from build123d import *

# Parameters (mm, degrees)
SKETCH1_W           = 135
SKETCH1_H           = 80
BOSS_EXTRUDE1_DEPTH = 40
SKETCH2_R           = 1.5
CUT_EXTRUDE1_DEPTH  = 10
SKETCH3_R           = 1.5
CUT_EXTRUDE2_DEPTH  = 10
CAVITY1_START       = 5.91875
CAVITY1_DEPTH       = 68.1625
CAVITY1_START_2     = 5
CAVITY1_2_DEPTH     = 125
SKETCH4_W           = 135
SKETCH4_H           = 25
CUT_EXTRUDE3_DEPTH  = 100


with BuildPart() as part:
    # Sketch1 → Boss-Extrude1 (new body)
    with BuildSketch(Plane.XY):
        with Locations((67.5, 40)):
            Rectangle(SKETCH1_W, SKETCH1_H)
    extrude(amount=-BOSS_EXTRUDE1_DEPTH)

    # Sketch2 → Cut-Extrude1 (cut)
    with BuildSketch(Plane(origin=(0, 0, -40), x_dir=(-1, 0, 0), z_dir=(0, 0, -1))):
        with Locations((-53.3, 40)):
            Circle(SKETCH2_R)
        with Locations((-53.3, 58.35)):
            Circle(SKETCH2_R)
        with Locations((-53.3, 21.65)):
            Circle(SKETCH2_R)
        with Locations((-23.3, 58.35)):
            Circle(SKETCH2_R)
        with Locations((-23.3, 40)):
            Circle(SKETCH2_R)
        with Locations((-23.3, 21.65)):
            Circle(SKETCH2_R)
        with Locations((-115.7, 40)):
            Circle(SKETCH2_R)
        with Locations((-115.7, 56)):
            Circle(SKETCH2_R)
        with Locations((-113.1, 61.75)):
            Circle(SKETCH2_R)
        with Locations((-113.1, 49.75)):
            Circle(SKETCH2_R)
        with Locations((-113.1, 18.25)):
            Circle(SKETCH2_R)
        with Locations((-113.1, 30.25)):
            Circle(SKETCH2_R)
    extrude(amount=-CUT_EXTRUDE1_DEPTH, mode=Mode.SUBTRACT)

    # Sketch3 → Cut-Extrude2 (cut)
    with BuildSketch(Plane.ZY):
        with Locations((-10, 54.05)):
            Circle(SKETCH3_R)
        with Locations((-10, 25.95)):
            Circle(SKETCH3_R)
        with Locations((-26, 40)):
            Circle(SKETCH3_R)
    extrude(amount=-CUT_EXTRUDE2_DEPTH, mode=Mode.SUBTRACT)

    # Cavity1: read off the stored shape, not the designer's step
    # Cavity1 outline → Cavity1 (cut)
    with BuildSketch(Plane(origin=(0, 0, 0), x_dir=(1, 0, 0), z_dir=(0, 1, 0)).offset(CAVITY1_START)):
        Polygon((128.3771626, 35.7), (6.6228374, 35.7), (5.688, 0), (129.312, 0), align=None)
    extrude(amount=CAVITY1_DEPTH, mode=Mode.SUBTRACT)

    # Cavity1 2 outline → Cavity1 2 (add)
    with BuildSketch(Plane.YZ.offset(CAVITY1_START_2)):
        Polygon((74.08125, 0), (73.141830064, -35.7), (74.08125, -35.7), align=None)
        Polygon((6.858169936, -35.7), (5.91875, 0), (5.91875, -35.7), align=None)
    extrude(amount=CAVITY1_2_DEPTH)

    # Sketch4 → Cut-Extrude3 (cut)
    with BuildSketch(Plane(origin=(0, 80, 0), x_dir=(1, 0, 0), z_dir=(0, 1, 0))):
        with Locations((67.5, 12.5)):
            Rectangle(SKETCH4_W, SKETCH4_H)
    extrude(amount=-CUT_EXTRUDE3_DEPTH, mode=Mode.SUBTRACT)


solid = part.part
Work out the finished part from the listing and answer in its coordinate system (mm). A direction names the side the tool comes from. Round coordinates to 2 decimals unless told otherwise and drop trailing zeros. Write each loop counter-clockwise with the first axis right and the second up, starting at its lowest first coordinate (ties: lowest second). Pieces come first, ordered by that corner, then holes.
1) A tool of negligible diameter and unlimited length cuts with its end or side. For faces 5 (the cylindrical face through (112.41, 48.42, -37.88)), 6 (the flat face through (68, 40, -35.7)), from which of +Z, -Z, +X, -X, +Y, -Y can it reach the whole face along a straight path? Write none if from no direction.
2) Given pin 1 Ø8 at (x, y) = (14, 30.5) entering from +Z, flat-ended and moving along its own axis, determine where the tip first touches the part or whether it passes through.
3) A cutting plane is placed at C-C (z = -30.25). Give the vertices of the cut face in (x, y).
4) Straight lines are drawn through the part: line 1 (Y direction, x = 115.7, z = -38.55); line 2 (Y direction, x = 23.3, z = -38.6); line 3 (Y direction, x = 113.1, z = -38.3). For each, find the intervals that lie inside material, in ascending order.
5) The mould has two halves that part along Z. Classify faces 1 (the flat face through (67, 5, -25)), 2 (the cylindrical face through (114.314, 39.425, -37.88)), 3 (the cylindrical face through (3.2, 40, -27.5)), 4 (the flat face through (67, 41, -40)): pulls with the +Z half, pulls with the -Z half, needs draft (parallel to the pull), parting line crosses it, or undercut.
6) A cutting plane is placed at B-B (x = 23.3). Give the vertices of the cut face in (y, z), plus the area to 3 significant figures.
7) A cutting plane is placed at D-D (x = 121.5). Give the vertices of the cut face in (y, z), plus the area to 3 significant figures.
8) A cutting plane is placed at A-A (y = 30.25). Give the vertices of the cut face in (x, z), plus the area to 3 significant figures.
Completed:
1. face 5: +Z, -Z
1. face 6: +Z
2. pin 1: stops at z = -35.7
3. outline: (0, 0) - (135, 0) - (135, 80) - (0, 80) - close; hole (6.48, 6.71) - (128.52, 6.71) - (128.52, 73.29) - (6.48, 73.29) - close
4. line 1: y = 0 to 38.5, 41.5 to 54.5, 57.5 to 80
4. line 2: y = 0 to 20.15, 23.15 to 38.5, 41.5 to 56.85, 59.85 to 80
4. line 3: y = 0 to 16.75, 19.75 to 28.75, 31.75 to 48.25, 51.25 to 60.25, 63.25 to 80
5. face 1: pulls with the +Z half
5. face 2: needs draft
5. face 3: undercut
5. face 4: pulls with the -Z half
6. outline: (0, -40) - (20.15, -40) - (20.15, -35.7) - (6.86, -35.7) - (6.58, -25) - (0, -25) - close; (23.15, -40) - (38.5, -40) - (38.5, -35.7) - (23.15, -35.7) - close; (41.5, -40) - (56.85, -40) - (56.85, -35.7) - (41.5, -35.7) - close; (59.85, -40) - (80, -40) - (80, -25) - (73.42, -25) - (73.14, -35.7) - (59.85, -35.7) - close
6. area: 449 mm2
7. outline: (0, -40) - (80, -40) - (80, -25) - (73.42, -25) - (73.14, -35.7) - (6.86, -35.7) - (6.58, -25) - (0, -25) - close
7. area: 488 mm2
8. outline: (0, -40) - (111.6, -40) - (111.6, -35.7) - (6.62, -35.7) - (6.34, -25) - (0, -25) - close; (114.6, -40) - (135, -40) - (135, -25) - (128.66, -25) - (128.38, -35.7) - (114.6, -35.7) - close
8. area: 706 mm2
